Answer from the drawing. Dimensions are ordinates in mm from the lowest x, y and z of the part. Coordinates: 2 decimals unless noted, no trailing zeros. Write each loop counter-clockwise with the first axis right and the second up, starting at its lowest first coordinate (ties: lowest second). Pieces come first, ordered by that corner, then holes.
(1) Given pin 1 (1.7 mm diameter, centred on x = 35, y = 5, fed in from +Z), flat-ended and moving along its own axis, determine where the tip first touches the part or whether it passes through.
(2) Section A-A on x = 25.5 is taken. Write down the section's boundary in (y, z), then the cut area to 4 significant figures.
(3) Section D-D on x = 5 is taken. Write down the section's boundary in (y, z).
(4) Find the intervals of material crossed by probe 1 along X at (y, z) = (5, 0.75); probe 2 along Y at (x, z) = (35, 1.1); probe 3 along Y at (x, z) = (25.5, 0.85), in increasing order.
(5) Section C-C on z = 0.9 is taken. Write down the section's boundary in (x, y).
(6) Section B-B on y = 5 is taken. Write down the section's boundary in (x, z), then the cut area to 3 significant figures.
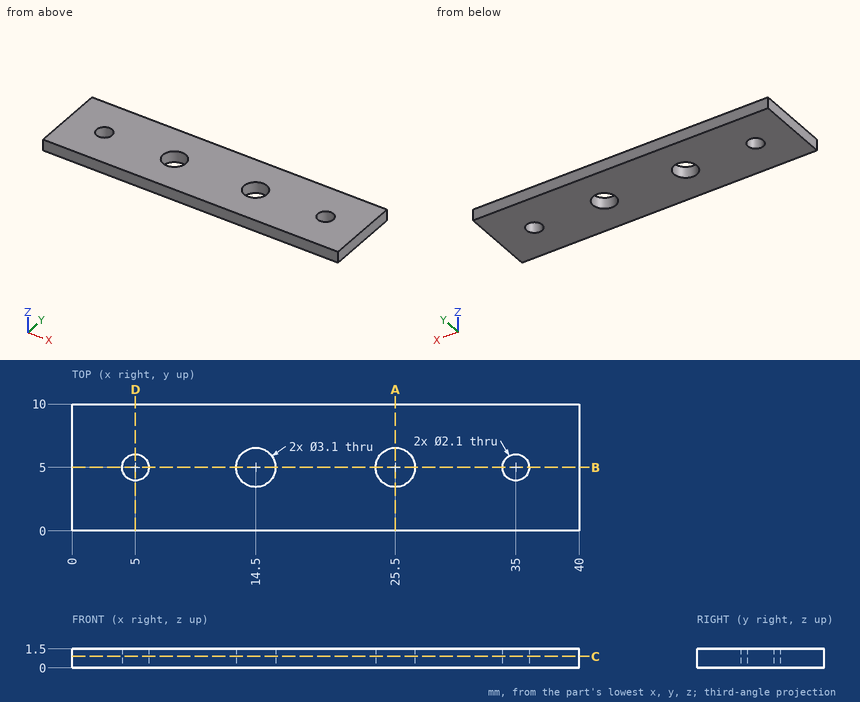
Response:
1. pin 1: passes through
2. outline: (0, 0) - (3.45, 0) - (3.45, 1.5) - (0, 1.5) - close; (6.55, 0) - (10, 0) - (10, 1.5) - (6.55, 1.5) - close
2. area: 10.35 mm2
3. outline: (0, 0) - (3.95, 0) - (3.95, 1.5) - (0, 1.5) - close; (6.05, 0) - (10, 0) - (10, 1.5) - (6.05, 1.5) - close
4. probe 1: x = 0 to 3.95, 6.05 to 12.95, 16.05 to 23.95, 27.05 to 33.95, 36.05 to 40
4. probe 2: y = 0 to 3.95, 6.05 to 10
4. probe 3: y = 0 to 3.45, 6.55 to 10
5. outline: (0, 0) - (40, 0) - (40, 10) - (0, 10) - close; hole circle Ø2.1 at (5, 5); hole circle Ø3.1 at (14.5, 5); hole circle Ø3.1 at (25.5, 5); hole circle Ø2.1 at (35, 5)
6. outline: (0, 0) - (3.95, 0) - (3.95, 1.5) - (0, 1.5) - close; (6.05, 0) - (12.95, 0) - (12.95, 1.5) - (6.05, 1.5) - close; (16.05, 0) - (23.95, 0) - (23.95, 1.5) - (16.05, 1.5) - close; (27.05, 0) - (33.95, 0) - (33.95, 1.5) - (27.05, 1.5) - close; (36.05, 0) - (40, 0) - (40, 1.5) - (36.05, 1.5) - close
6. area: 44.4 mm2
